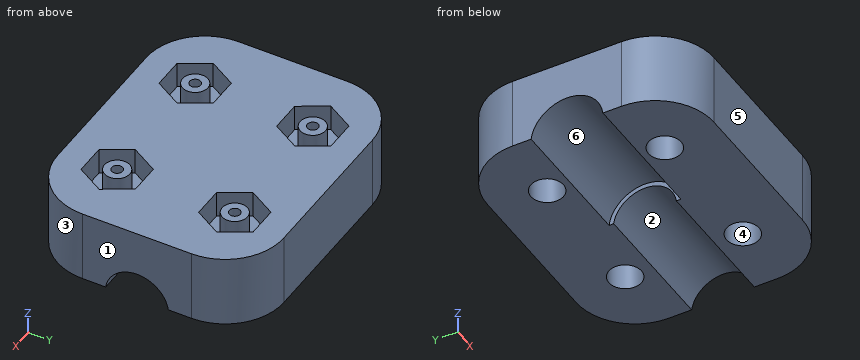
```python
from build123d import *

# Parameters (mm, degrees)
BOSS_EXTRUDE2_DEPTH = 8
SKETCH10_R          = 1.800000439
CUT_EXTRUDE5_DEPTH  = 4.7
CUT_EXTRUDE6_DEPTH  = 2.9
SKETCH12_R          = 3.5
CUT_EXTRUDE7_DEPTH  = 31
SKETCH13_R          = 4
CUT_EXTRUDE8_DEPTH  = 15
SKETCH14_R          = 1.402200439
SKETCH14_R_2        = 0.606600439
BOSS_EXTRUDE3_DEPTH = 2.9


with BuildPart() as part:
    # Sketch9 → Boss-Extrude2 (new body)
    with BuildSketch(Plane.XY):
        with BuildLine():
            Line((15, -20.019238), (15, -7.980762))
            ThreePointArc((15, -7.980762), (13.101828757, -3.398171243), (8.519238, -1.5))
            Line((8.519238, -1.5), (-8.519238, -1.5))
            ThreePointArc((-8.519238, -1.5), (-13.101828757, -3.398171243), (-15, -7.980762))
            Line((-15, -7.980762), (-15, -20.019238))
            ThreePointArc((-15, -20.019238), (-13.101828757, -24.601828757), (-8.519238, -26.5))
            Line((-8.519238, -26.5), (8.519238, -26.5))
            ThreePointArc((8.519238, -26.5), (13.101828757, -24.601828757), (15, -20.019238))
        make_face()
    extrude(amount=-BOSS_EXTRUDE2_DEPTH)

    # Sketch10 → Cut-Extrude5 (cut)
    with BuildSketch(Plane(origin=(0, 0, -8), x_dir=(-1, 0, 0), z_dir=(0, 0, -1))):
        with Locations((-7.499999289, -7.499999745)):
            Circle(SKETCH10_R)
        with Locations((7.499999289, -7.499999745)):
            Circle(SKETCH10_R)
        with Locations((7.499999289, -20.500000255)):
            Circle(SKETCH10_R)
        with Locations((-7.499999289, -20.500000255)):
            Circle(SKETCH10_R)
    extrude(amount=-CUT_EXTRUDE5_DEPTH, mode=Mode.SUBTRACT)

    # Sketch11 → Cut-Extrude6 (cut)
    with BuildSketch(Plane.XY):
        Polygon((9.232050097, -4.499999745), (10.964100904, -7.499999745), (9.232050097, -10.499999745), (5.767948482, -10.499999745), (4.035897674, -7.499999745), (5.767948482, -4.499999745), align=None)
        Polygon((-9.232050097, -23.500000255), (-10.964100904, -20.500000255), (-9.232050097, -17.500000255), (-5.767948482, -17.500000255), (-4.035897674, -20.500000255), (-5.767948482, -23.500000255), align=None)
        Polygon((10.964100904, -20.500000255), (9.232050097, -17.500000255), (5.767948482, -17.500000255), (4.035897674, -20.500000255), (5.767948482, -23.500000255), (9.232050097, -23.500000255), align=None)
        Polygon((-10.964100904, -7.499999745), (-9.232050097, -10.499999745), (-5.767948482, -10.499999745), (-4.035897674, -7.499999745), (-5.767948482, -4.499999745), (-9.232050097, -4.499999745), align=None)
    extrude(amount=-CUT_EXTRUDE6_DEPTH, mode=Mode.SUBTRACT)

    # Sketch12 → Cut-Extrude7 (cut, through all)
    with BuildSketch(Plane(origin=(15, 0, 0), x_dir=(0, 0, -1), z_dir=(1, 0, 0))):
        with Locations((8.499999447, -14)):
            Circle(SKETCH12_R)
    extrude(amount=-CUT_EXTRUDE7_DEPTH, mode=Mode.SUBTRACT)

    # Sketch13 → Cut-Extrude8 (cut)
    with BuildSketch(Plane.ZY.offset(15)):
        with Locations((-8.499999973, -14)):
            Circle(SKETCH13_R)
    extrude(amount=-CUT_EXTRUDE8_DEPTH, mode=Mode.SUBTRACT)

    # Sketch14 → Boss-Extrude3 (add)
    with BuildSketch(Plane.XY.offset(-2.9)):
        with Locations((-7.499999289, -7.499999745)):
            Circle(SKETCH14_R)
        with Locations((-7.499999289, -7.499999745)):
            Circle(SKETCH14_R_2, mode=Mode.SUBTRACT)
        with Locations((7.499999289, -7.499999745)):
            Circle(SKETCH14_R)
        with Locations((7.499999289, -7.499999745)):
            Circle(SKETCH14_R_2, mode=Mode.SUBTRACT)
        with Locations((-7.499999289, -20.500000255)):
            Circle(SKETCH14_R)
        with Locations((-7.499999289, -20.500000255)):
            Circle(SKETCH14_R_2, mode=Mode.SUBTRACT)
        with Locations((7.499999289, -20.500000255)):
            Circle(SKETCH14_R)
        with Locations((7.499999289, -20.500000255)):
            Circle(SKETCH14_R_2, mode=Mode.SUBTRACT)
    extrude(amount=BOSS_EXTRUDE3_DEPTH)


solid = part.part
```
CAD build for the part. Positions are in the model's coordinates, mm. Face numbers are marked on the shaded views. A direction names the side the tool comes from. Coordinates: 2 decimals unless noted, no trailing zeros. Write each loop counter-clockwise with the first axis right and the second up, starting at its lowest first coordinate (ties: lowest second). Pieces come first, ordered by that corner, then holes. Notation, with made-up numbers: (58, -34) -> (102, -34) arc R28 ccw to (102, -1) -> close; hole circle Ø8 at (1, 73). An arc over 180 degrees is marked (long way). Return JSON: item names as keys, results as strings. Group by question number.
Q1. Cut at A-A, the plane z = -2.5. State how many separate pieces and enclosed holes the cut face has, then the cut area to 3 significant figures.
Q2. Cut at D-D, the plane x = -12. Give the cut face in (y, z).
Q3. Cut at B-B, the plane x = -2.5. Give the cut face in (y, z).
Q4. Flat gauge pins, fed straight in: pin 1 (1.5 mm diameter, centred on y = -4, z = -1.5, fed in from -X); pin 2 (1.3 mm diameter, centred on x = -7.5, y = -20.5, fed in from +Z); pin 3 (1.5 mm diameter, centred on y = -22.5, z = -6.5, fed in from +X); pin 4 (1 mm diameter, centred on x = 7.5, y = -20.5, fed in from +Z). Where does each tip first touch, or does it go through?
Q5. Pull direction Y, two halves, no side cores. Call the marked faces 1, 2 and 3: released by +Y, released by -Y, zero draft, split by the parting line, or undercut.
Q6. Which spindle directions (+Z, -Z, +X, -X, +Y, -Y) get a long thin tool onto all of the face, cutting with end or side? Do the marked faces 4, 5 and 6. Say none if no direction does.
Q7. Drill centre lines: line 1 (Y direction, x = 7.5, z = -4.8); line 2 (Y direction, x = -7.5, z = -5.9); line 3 (X direction, y = -20.5, z = -4.45). Where is each one in solid material? Low to high.
Q8. Cut at C-C, the plane y = -19.5. Give the cut face in (x, z).
Returned:
{
 "1": {"separate pieces": "5", "enclosed holes": "8", "area": "609 mm2"},
 "2": {"outline": "(-25.49, -8) -> (-17.97, -8) arc R4 cw to (-10.03, -8) -> (-2.51, -8) -> (-2.51, 0) -> (-25.49, 0) -> close"},
 "3": {"outline": "(-26.5, -8) -> (-17.97, -8) arc R4 cw to (-10.03, -8) -> (-1.5, -8) -> (-1.5, 0) -> (-26.5, 0) -> close"},
 "4": {"pin 1": "stops at x = -14.14", "pin 2": "stops at z = 0", "pin 3": "stops at x = 14.76", "pin 4": "stops at z = -2.9"},
 "5": {"face 1": "zero draft", "face 2": "undercut", "face 3": "released by -Y"},
 "6": {"face 4": "-Z", "face 5": "+Z, -Z, +X, -X, -Y", "face 6": "-Z, -X"},
 "7": {"line 1": "y = -26.5 to -22.3, -18.7 to -9.3, -5.7 to -1.5", "line 2": "y = -26.5 to -22.3, -18.7 to -17.04, -10.96 to -9.3, -5.7 to -1.5", "line 3": "x = -14.98 to -9.3, -5.7 to 5.7, 9.3 to 14.98"},
 "8": {"outline": "(-15, -8) -> (-9, -8) -> (-9, -3.3) -> (-6, -3.3) -> (-6, -8) -> (6, -8) -> (6, -3.3) -> (9, -3.3) -> (9, -8) -> (15, -8) -> (15, 0) -> (10.39, 0) -> (10.39, -2.9) -> (8.48, -2.9) -> (8.48, 0) -> (6.52, 0) -> (6.52, -2.9) -> (4.61, -2.9) -> (4.61, 0) -> (-4.61, 0) -> (-4.61, -2.9) -> (-6.52, -2.9) -> (-6.52, 0) -> (-8.48, 0) -> (-8.48, -2.9) -> (-10.39, -2.9) -> (-10.39, 0) -> (-15, 0) -> close"}
}
